Build history of the part. All positions in model axes, mm. Give positions to 0.01 mm unless a question says otherwise; leave off trailing zeros. Order: outer loops, then holes, each group sorted by start corner. A loop starts at its lowest first (then second) coordinate and runs counter-clockwise, first axis right, second up. Notation, with made-up numbers: (35.5, 24) - (58.5, 24) arc R28 cw to (58.5, 53) - close; hole circle Ø1 at (-5.5, 84.5). An arc over 180 degrees is marked (long way). Use a Markdown table: item, result.
from build123d import *

# Parameters (mm, degrees)
SKETCH1_W            = 961
SKETCH1_H            = 790
SKETCH1_W_2          = 500
SKETCH1_H_2          = 150
BASE_FLANGE1_DEPTH   = 1.5
CUT_EXTRUDE1_REACH   = 926.653
SKETCH2_W            = 148
SKETCH2_H            = 60
CUT_EXTRUDE2_REACH   = 926.653
SKETCH3_W            = 600
SKETCH3_H            = 410
M3_CLEARANCE_HOLE1_D = 3.4
FILLET1_R            = 10
FILLET2_R            = 2


# Sheet-metal steps are written as plain solids
with BuildPart() as part:
    # Sketch1 → Base-Flange1 (new body)
    with BuildSketch(Plane.XY):
        with Locations((0, 395)):
            Rectangle(SKETCH1_W, SKETCH1_H)
        with Locations((0, 645)):
            Rectangle(SKETCH1_W_2, SKETCH1_H_2, mode=Mode.SUBTRACT)
    extrude(amount=-BASE_FLANGE1_DEPTH)

    # Sketch2 → Cut-Extrude1 (cut, up to next)
    with BuildSketch(Plane.XY, mode=Mode.PRIVATE) as cut_extrude1_sk1:
        with Locations((-406.5, 760)):
            Rectangle(SKETCH2_W, SKETCH2_H)
    cut_extrude1_tool1 = extrude(cut_extrude1_sk1.sketch, amount=-CUT_EXTRUDE1_REACH, mode=Mode.PRIVATE) & part.part
    cut_extrude1 = cut_extrude1_tool1.solids().sort_by_distance((-406.5, 760, 0))[0]
    add(cut_extrude1, mode=Mode.SUBTRACT)

    # Mirror1: Cut-Extrude1 across plane
    add(cut_extrude1.mirror(Plane(origin=(0, 0, 0), x_dir=(0, 0, 1), z_dir=(1, 0, 0))), mode=Mode.SUBTRACT)

    # Sketch3 → Cut-Extrude2 (cut, up to next)
    with BuildSketch(Plane(origin=(0, 0, -1.5), x_dir=(-1, 0, 0), z_dir=(0, 0, -1)), mode=Mode.PRIVATE) as cut_extrude2_sk1:
        with Locations((0, 285)):
            Rectangle(SKETCH3_W, SKETCH3_H)
    cut_extrude2_tool1 = extrude(cut_extrude2_sk1.sketch, amount=-CUT_EXTRUDE2_REACH, mode=Mode.PRIVATE) & part.part
    add(cut_extrude2_tool1.solids().sort_by_distance((0, 285, -1.5))[0], mode=Mode.SUBTRACT)

    # M3 Clearance Hole1 (through all)
    with Locations(Plane(origin=(0, 0, -1.5), x_dir=(-1, 0, 0), z_dir=(0, 0, -1))):
        with Locations((-315, 125), (-315, 149), (-315, 445), (-315, 421)):
            m3_clearance_hole1 = Hole(M3_CLEARANCE_HOLE1_D / 2)

    # Mirror2: M3 Clearance Hole1 across plane
    add(m3_clearance_hole1.mirror(Plane(origin=(0, 0, 0), x_dir=(0, 0, 1), z_dir=(1, 0, 0))), mode=Mode.SUBTRACT)

    # Fillet1
    fillet1_edges = [part.edges().sort_by_distance(p)[0] for p in [
        (-250, 720, -0.75),
        (250, 720, -0.75),
        (250, 570, -0.75),
        (-250, 570, -0.75),
        (-300, 490, -0.75),
        (-300, 80, -0.75),
        (300, 80, -0.75),
        (300, 490, -0.75),
    ]]
    fillet(fillet1_edges, radius=FILLET1_R)

    # Fillet2
    fillet2_edges = [part.edges().sort_by_distance(p)[0] for p in [
        (-480.5, 730, -0.75),
        (-332.5, 790, -0.75),
        (-332.5, 730, -0.75),
        (480.5, 730, -0.75),
        (332.5, 730, -0.75),
        (332.5, 790, -0.75),
        (480.5, 0, -0.75),
        (-480.5, 0, -0.75),
    ]]
    fillet(fillet2_edges, radius=FILLET2_R)


solid = part.part
1) Wall check: line 1 (Y direction, x = -240, z = -0.55); line 2 (Y direction, x = 315, z = -0.85); line 3 (X direction, y = 149, z = -0.35). Give the ranges that are in metal, low to high. Write a range as from..to.
Computed:
| item | result |
|---|---|
| line 1 | y = 0..80, 490..570, 720..790 |
| line 2 | y = 0..123.3, 126.7..147.3, 150.7..419.3, 422.7..443.3, 446.7..790 |
| line 3 | x = -480.5..-316.7, -313.3..-300, 300..313.3, 316.7..480.5 |
2) Pin check, flat tip, straight feed: P1, Ø4, axis at x = 315, y = 445, coming from the +Z side. Stop position of the tip, or through.
Computed:
| item | result |
|---|---|
| P1 | stops at z = 0 |
3) Slice it at B-B (x = -191). Write the cut outline in (y, z), and give its area (3 significant figures).
Computed:
| item | result |
|---|---|
| outline | (0, -1.5) - (80, -1.5) - (80, 0) - (0, 0) - close; (490, -1.5) - (570, -1.5) - (570, 0) - (490, 0) - close; (720, -1.5) - (790, -1.5) - (790, 0) - (720, 0) - close |
| area | 345 mm² |
4) Slice it at D-D (x = -383.5). Write the cut outline in (y, z), and give its area (4 significant figures).
Computed:
| item | result |
|---|---|
| outline | (0, -1.5) - (730, -1.5) - (730, 0) - (0, 0) - close |
| area | 1,095 mm² |
5) Slice it at C-C (z = -0.3). State how many separate pieces and enclosed holes the cut face has, and give its area (3 significant figures).
Computed:
| item | result |
|---|---|
| separate pieces | 1 |
| enclosed holes | 10 |
| area | 421,000 mm² |
6) Slice it at A-A (y = 269.5). Write the cut outline in (x, z).
Computed:
| item | result |
|---|---|
| outline | (-480.5, -1.5) - (-300, -1.5) - (-300, 0) - (-480.5, 0) - close; (300, -1.5) - (480.5, -1.5) - (480.5, 0) - (300, 0) - close |
